Autodesk Inventor part; units mm, degrees
ref_plane "Work Plane1" through (0, 0, 0.127) normal (0, 0, 1) x (1, 0, 0)
ref_plane "YZ Plane" through (0, 0, 0) normal (1, 0, 0) x (0, 1, 0)
ref_plane "XZ Plane" through (0, 0, 0) normal (0, 1, 0) x (-1, 0, 0)
sketch "Sketch1" plane through (0, 0, 0) normal (0, 0, 1) x (1, 0, 0)
  line L0 (21.0589, 9.4901) -> (21.0589, 9.4901)
  line L1 (21.6939, 8.8551) -> (21.6939, -0.0349)
  line L2 (21.0589, -0.6699) -> (21.0589, -0.6699)
  line L3 (20.4239, -0.0349) -> (20.4239, 8.8551)
  arc A0 (21.0589, 9.4901) -> (20.4239, 8.8551) centre (21.0589, 8.8551) ccw
  arc A1 (21.6939, 8.8551) -> (21.0589, 9.4901) centre (21.0589, 8.8551) ccw
  arc A2 (21.0589, -0.6699) -> (21.6939, -0.0349) centre (21.0589, -0.0349) ccw
  arc A3 (20.4239, -0.0349) -> (21.0589, -0.6699) centre (21.0589, -0.0349) ccw
  point P0 (0, 0)
  point P1 (21.6939, -0.6699)
  point P2 (21.6939, 9.4901)
  point P3 (20.4239, -0.6699)
  dimension "d0" = 1.27
  dimension "d1" = 10.16
  dimension "d2" = 0.635
extrude "Extrusion1" add sketch "Sketch1" along normal mid plane 0.762
sketch "Sketch2" plane through (0, 0, 0) normal (0, 0, 1) x (1, 0, 0)
  arc A0 (21.6939, 8.8551) -> (20.4239, 8.8551) centre (21.0589, 8.8551) ccw
  line L0 (20.4239, 8.8551) -> (20.4239, -0.0349)
  line L1 (21.6939, -0.0349) -> (21.6939, 8.8551)
  circle A1 centre (21.0589, 8.8551) radius 0.0635
  arc A2 (21.6939, 8.8551) -> (20.4239, 8.8551) centre (21.0589, 8.8551) ccw
  line L2 (20.4239, 4.1124) -> (21.6939, 4.1124)
  line L3 (21.6939, 8.8551) -> (21.6939, -0.0349)
  point P0 (0, 0)
  point P1 (20.4239, 8.8551)
  dimension "d5" = 0.127
extrude "Extrusion2" cut sketch "Sketch2" along normal mid plane 0.254
ref_plane "Work Plane1" through (0, 0, 0.127) normal (0, 0, 1) x (1, 0, 0)
sketch "Sketch4" plane through (0, 0, 0.127) normal (0, 0, 1) x (1, 0, 0)
  arc A0 (20.4239, -0.0349) -> (21.6939, -0.0349) centre (21.0589, -0.0349) ccw
  circle A1 centre (21.0589, -0.0349) radius 0.0127
  point P0 (0, 0)
  dimension "d11" = 0.0254
extrude "Extrusion4" cut sketch "Sketch4" along normal mid plane 1.8415
properties part number "body parts" material "PVC-Piping"
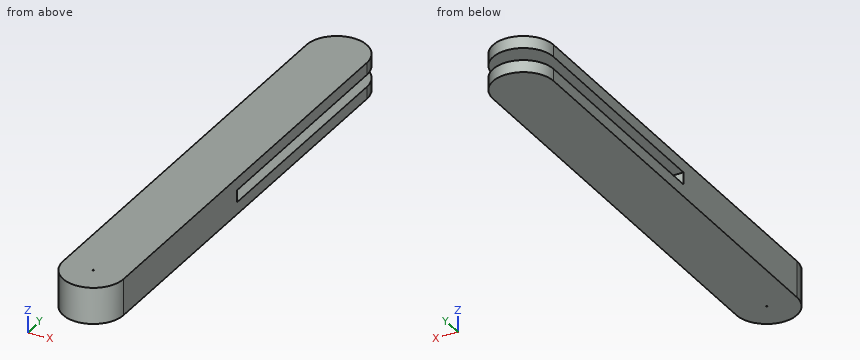
Could you check a few things on this model? Use its own coordinates, in mm. Coordinates: 2 decimals unless noted, no trailing zeros. Write each loop counter-clockwise with the first axis right and the second up, starting at its lowest first coordinate (ties: lowest second). Pieces come first, ordered by that corner, then holes. Notation, with made-up numbers: (29, 18.25) -> (65, 18.25) arc R28 ccw to (65, 52.25) -> close; hole circle Ø9 at (69, 23.25). An arc over 180 degrees is marked (long way). One line per question, with ' | ' between items. Start each with the question number.
1. If we section it at B-B (y = 7.5): Please give me the cut outline in (x, z).
2. Please list where these lines run through material, in increasing order: line 1 along Z through (x, y) = (21.3, 5.5); line 2 along Y through (x, z) = (21.2, 0.2); line 3 along Y through (x, z) = (21.45, -0.2).
3. If we section it at A-A (z = 0): Please give me the cut outline in (x, y) (1 decimal).
4. If we section it at D-D (x = 21.25): Please give me the cut outline in (y, z), and give its area (3 significant figures).
5. If we section it at C-C (x = 20.6): Please give me the cut outline in (y, z), and give its area (3 significant figures).
Return value:
1) outline: (20.42, -0.38) -> (21.69, -0.38) -> (21.69, -0.13) -> (20.42, -0.13) -> close; (20.42, 0.13) -> (21.69, 0.13) -> (21.69, 0.38) -> (20.42, 0.38) -> close
2) line 1: z = -0.38 to -0.13, 0.13 to 0.38 | line 2: y = -0.65 to 9.47 | line 3: y = -0.54 to 9.36
3) outline: (20.4, 0) arc R0.6 ccw to (21.7, 0) -> (21.7, 4.1) -> (20.4, 4.1) -> close; circle Ø0.1 at (21.1, 8.9); hole circle Ø0 at (21.1, 0)
4) outline: (-0.64, -0.38) -> (9.46, -0.38) -> (9.46, -0.13) -> (4.11, -0.13) -> (4.11, 0.13) -> (9.46, 0.13) -> (9.46, 0.38) -> (-0.64, 0.38) -> close | area: 6.34 mm²
5) outline: (-0.47, -0.38) -> (9.29, -0.38) -> (9.29, -0.13) -> (4.11, -0.13) -> (4.11, 0.13) -> (9.29, 0.13) -> (9.29, 0.38) -> (-0.47, 0.38) -> close | area: 6.13 mm²
